Here's the drawing with two shaded views (mm, measured from the low corner). I have some questions. Coordinates: 2 decimals unless noted, no trailing zeros. Loops run counter-clockwise (first coordinate to the right, second up) from the corner with the lowest first, then second, coordinate; pieces in that order, holes last. Notation, with made-up numbers: (-11, 24.25) -> (2, 24.25) arc R23 cw to (2, 59.25) -> close; hole circle Ø7 at (75, 79.25). An arc over 180 degrees is marked (long way). Answer as a JSON object with one key per item and string values. Group by question number.
Q1. I want a section at D-D on y = 4. Write out the boundary of the cut face in (x, z), then the cut area to 3 significant figures.
Q2. I want a section at A-A on x = 4.25. Write out the boundary of the cut face in (y, z) (3 decimals), then the cut area to 3 significant figures.
Q3. I'm going to push a flat-ended pin straight in: pin 1 (2 mm diameter, centred on x = 1.5, y = 7, fed in from -Z). Where does the tip first touch, or does it pass through?
Q4. I need wall thicknesses on line 1 (Y direction, x = 1.25, z = 18) (3 decimals); line 2 (Z direction, x = 7.25, y = 10) (3 decimals); line 3 (Z direction, x = 1.5, y = 11.25). Which ranges of each line are inside material? Lowest first, please.
Q5. I want a section at B-B on y = 7.5. Write out the boundary of the cut face in (x, z) (3 decimals).
Q6. I want a section at C-C on y = 18. Write out the boundary of the cut face in (x, z).
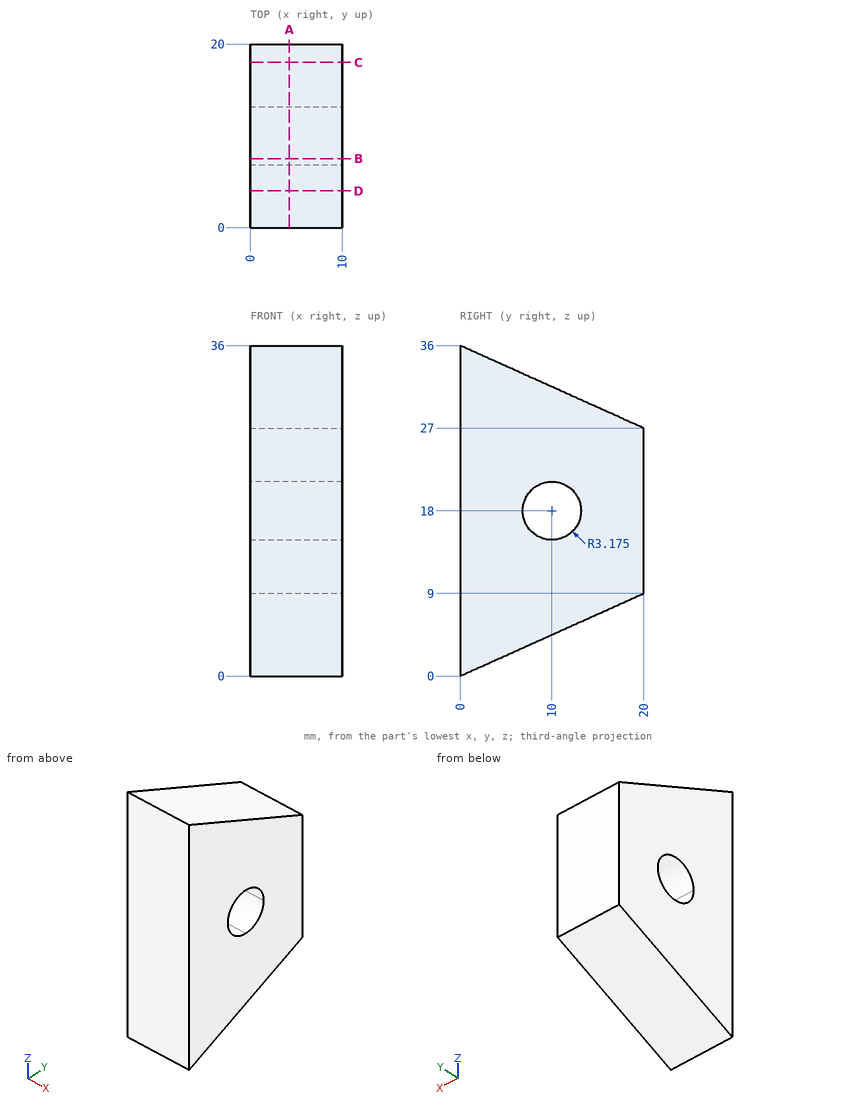
Result set:
{
 "1": {"outline": "(0, 1.8) -> (10, 1.8) -> (10, 34.2) -> (0, 34.2) -> close", "area": "324 mm²"},
 "2": {"outline": "(0, 0) -> (20, 9) -> (20, 27) -> (0, 36) -> close; hole circle Ø6.35 at (10, 18)", "area": "508 mm²"},
 "3": {"pin 1": "stops at z = 2.7"},
 "4": {"line 1": "y = 0 to 6.825, 13.175 to 20", "line 2": "z = 4.5 to 14.825, 21.175 to 31.5", "line 3": "z = 5.06 to 15.08, 20.92 to 30.94"},
 "5": {"outline": "(0, 3.375) -> (10, 3.375) -> (10, 16.043) -> (0, 16.043) -> close; (0, 19.957) -> (10, 19.957) -> (10, 32.625) -> (0, 32.625) -> close"},
 "6": {"outline": "(0, 8.1) -> (10, 8.1) -> (10, 27.9) -> (0, 27.9) -> close"}
}
